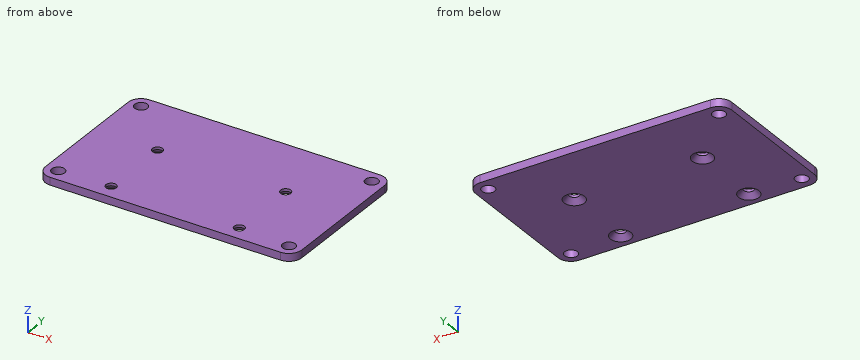
Autodesk Inventor part; units mm, degrees
ref_plane "YZ Plane" through (0, 0, 0) normal (1, 0, 0) x (0, 1, 0)
ref_plane "XZ Plane" through (0, 0, 0) normal (0, 1, 0) x (-1, 0, 0)
ref_plane "XY Plane" through (0, 0, 0) normal (0, 0, 1) x (1, 0, 0)
sketch "Sketch1" plane through (0, 0, 0) normal (0, 0, 1) x (1, 0, 0)
  line L0 (-50, -30) -> (50, -30)
  line L1 (50, -30) -> (50, 30)
  line L2 (50, 30) -> (-50, 30)
  line L3 (-50, 30) -> (-50, -30)
  line L4 (-50, -30) -> (50, 30) construction
  line L5 (50, -30) -> (-50, 30) construction
  point P0 (0, 0)
  dimension "d0" = 60
  dimension "d1" = 100
extrude "Plate1" add sketch "Sketch1" along normal blind 3
sketch "Sketch2" plane through (0, 0, 3) normal (0, 0, 1) x (1, 0, 0)
  line L0 (-50, -30) -> (-50, 30)
  line L1 (-50, 30) -> (50, 30)
  line L2 (50, -30) -> (-50, -30)
  line L3 (50, 30) -> (50, -30)
  point P0 (0, 0)
  point P1 (-45, 25)
  point P2 (45, 25)
  point P3 (45, -25)
  point P4 (-45, -25)
  dimension "d3" = 5
  dimension "d4" = 5
  dimension "d5" = 5
  dimension "d6" = 5
  dimension "d7" = 5
hole "Hole1" at (-45, 25, 3) at (45, 25, 3) at (45, -25, 3) at (-45, -25, 3) direction (0, 0, -1) diameter 5 depth 3
sketch "Sketch3" plane through (0, 0, 0) normal (0, 0, 1) x (1, 0, 0)
  line L0 (50, -30) -> (-50, -30)
  point P0 (0, 0)
  point P1 (-25, 4)
  point P2 (25, 4)
  point P3 (25, -24)
  point P4 (-25, -24)
  dimension "d15" = 28
  dimension "d16" = 6
  dimension "d17" = 50
  dimension "d18" = 25
hole "Hole2" at (-25, 4, 0) at (25, 4, 0) at (25, -24, 0) at (-25, -24, 0) direction (0, 0, 1) diameter 4 depth 3 countersink diameter 8 countersink angle 90
fillet "Fillet1" radius 5 4 edges at (-50, 30, 1.5) (-50, -30, 1.5) (50, -30, 1.5) (50, 30, 1.5)
equation "\"d13\" = Stärke"
equation "\"d2\" = Stärke"
equation "\"Biegeradius\" = Stärke"
equation "\"BreiteBiegungsfreistellung\" = Stärke"
equation "\"TiefeBiegungsfreistellung\" = 0.5 * Stärke"
equation "\"GrößeEckenfreistellung\" = 4 * Stärke"
equation "\"MinimalRest\" = 2 * Stärke"
equation "\"Übergangsradius\" = Biegeradius"
equation "\"JacobiRadiusGröße\" = Biegeradius"
equation "\"Abstandsgröße\" = Stärke"
properties part number "02"
Can you work these out from the model? Positions are in its coordinate system, mm. Give positions to 0.01 mm unless a question says otherwise; leave off trailing zeros. Loops run counter-clockwise (first coordinate to the right, second up) from the corner with the lowest first, then second, coordinate; pieces in that order, holes last. Notation, with made-up numbers: M 73,17 L 104,17 A16 ccw 104,27 Z; hole C -38.75,63 d3. An arc over 180 degrees is marked long. Answer in a Markdown table with one row per item.
1. For pin 1 Ø6.5 at (x, y) = (-25, 4) entering from -Z; pin 2 Ø8 at (x, y) = (45, -25) entering from +Z; pin 3 Ø5 at (x, y) = (-25, -24) entering from -Z; pin 4 Ø4.5 at (x, y) = (25, 4) entering from -Z, each with a flat end and sliding along its axis, tell me the tip position at first contact or that it passes through.
Taken from the geometry:
| item | result |
|---|---|
| pin 1 | stops at z = 0.75 |
| pin 2 | stops at z = 3 |
| pin 3 | stops at z = 1.5 |
| pin 4 | stops at z = 1.75 |
2. Suppose I cut it at A-A on x = -25. Write out the boundary of the cut face in (y, z), plus the area to 3 significant figures.
Taken from the geometry:
| item | result |
|---|---|
| outline | M -30,0 L -28,0 L -26,2 L -26,3 L -30,3 Z; M -22,2 L -20,0 L 0,0 L 2,2 L 2,3 L -22,3 Z; M 6,2 L 8,0 L 30,0 L 30,3 L 6,3 Z |
| area | 148 mm² |
3. Suppose I cut it at C-C on z = 1.55. Count the separate pieces of the cut face and the enclosed holes in it, plus the area to 3 significant figures.
Taken from the geometry:
| item | result |
|---|---|
| separate pieces | 1 |
| enclosed holes | 8 |
| area | 5,820 mm² |
4. Suppose I cut it at D-D on y = -24. Write out the boundary of the cut face in (x, z).
Taken from the geometry:
| item | result |
|---|---|
| outline | M -50,0 L -47.29,0 L -47.29,3 L -50,3 Z; M -42.71,0 L -29,0 L -27,2 L -27,3 L -42.71,3 Z; M -23,2 L -21,0 L 21,0 L 23,2 L 23,3 L -23,3 Z; M 27,2 L 29,0 L 42.71,0 L 42.71,3 L 27,3 Z; M 47.29,0 L 50,0 L 50,3 L 47.29,3 Z |
5. Suppose I cut it at B-B on y = 4. Write out the boundary of the cut face in (x, z).
Taken from the geometry:
| item | result |
|---|---|
| outline | M -50,0 L -29,0 L -27,2 L -27,3 L -50,3 Z; M -23,2 L -21,0 L 21,0 L 23,2 L 23,3 L -23,3 Z; M 27,2 L 29,0 L 50,0 L 50,3 L 27,3 Z |
6. If I drill on line 1 along Y through (x, z) = (25, 2.7); line 2 along Y through (x, z) = (45, 1.05); line 3 along X through (y, z) = (26, 2.85), over which ranges is the centre line in solid material (lowest first)?
Taken from the geometry:
| item | result |
|---|---|
| line 1 | y = -30 to -26, -22 to 2, 6 to 30 |
| line 2 | y = -30 to -27.5, -22.5 to 22.5, 27.5 to 30 |
| line 3 | x = -49.9 to -47.29, -42.71 to 42.71, 47.29 to 49.9 |
